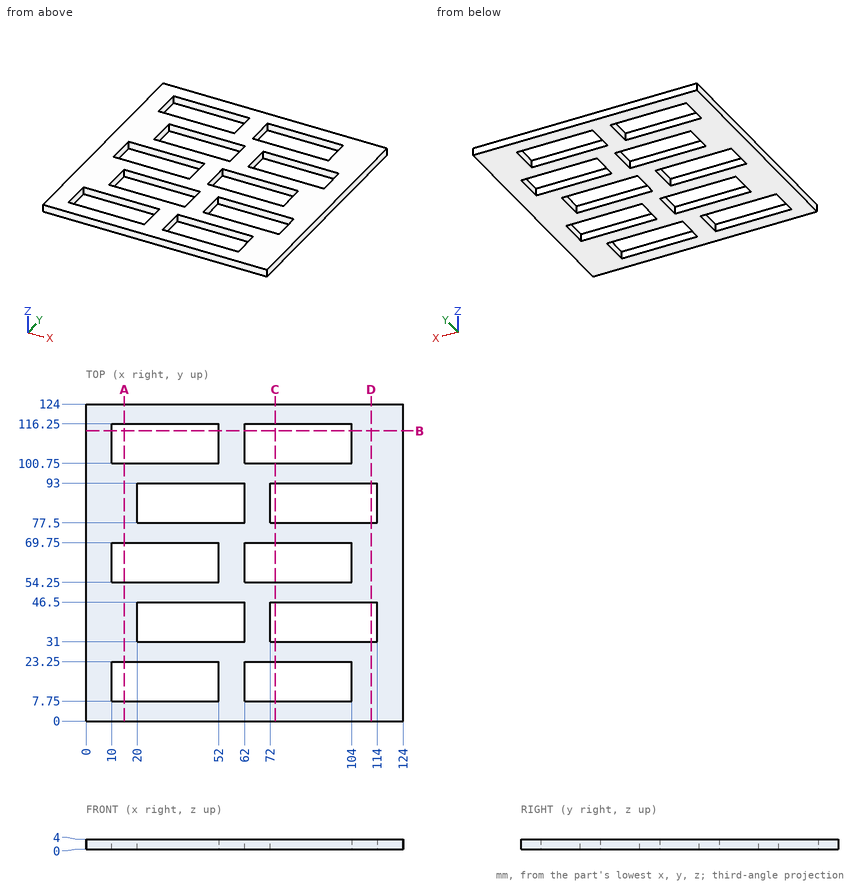
The figure shows three views and two pictorial views of one solid part (mm, origin at its lowest corner). Answer the questions. Coordinates: 2 decimals unless noted, no trailing zeros. Write each loop counter-clockwise with the first axis right and the second up, starting at its lowest first coordinate (ties: lowest second). Pieces come first, ordered by that corner, then holes. Notation, with made-up numbers: M 79.25,38.5 L 135.25,38.5 A21 ccw 135.25,76.5 Z; hole C 33,21.5 d10. An arc over 180 degrees is marked long. Answer as CSV lines item,"result". Start each with the question number.
Item 1: A flat-ended cylindrical pin translates along its axis: P1, Ø5, axis at x = 34, y = 103.5, coming from the +Z side. Find the tip coordinate at first contact, or state that the pin passes through.
Item 2: Section C-C on x = 74 is taken. Write down the section's boundary in (y, z), and give its area (3 significant figures).
Item 3: Section D-D on x = 111.5 is taken. Write down the section's boundary in (y, z), and give its area (3 significant figures).
Item 4: Section A-A on x = 15 is taken. Write down the section's boundary in (y, z).
Item 5: Consider L1, parallel to X at y = 34.5, z = 3.25; L2, parallel to Y at x = 19, z = 0.4; L3, parallel to X at y = 107, z = 1. Determine where each line is inside the solid, lowest interval first.
Item 6: Section B-B on y = 113.5 is taken. Write down the section's boundary in (x, z), and give its area (3 significant figures).
Checks:
1,P1,"passes through"
2,outline,"M 0,0 L 7.75,0 L 7.75,4 L 0,4 Z; M 23.25,0 L 31,0 L 31,4 L 23.25,4 Z; M 46.5,0 L 54.25,0 L 54.25,4 L 46.5,4 Z; M 69.75,0 L 77.5,0 L 77.5,4 L 69.75,4 Z; M 93,0 L 100.75,0 L 100.75,4 L 93,4 Z; M 116.25,0 L 124,0 L 124,4 L 116.25,4 Z"
2,area,"186 mm²"
3,outline,"M 0,0 L 31,0 L 31,4 L 0,4 Z; M 46.5,0 L 77.5,0 L 77.5,4 L 46.5,4 Z; M 93,0 L 124,0 L 124,4 L 93,4 Z"
3,area,"372 mm²"
4,outline,"M 0,0 L 7.75,0 L 7.75,4 L 0,4 Z; M 23.25,0 L 54.25,0 L 54.25,4 L 23.25,4 Z; M 69.75,0 L 100.75,0 L 100.75,4 L 69.75,4 Z; M 116.25,0 L 124,0 L 124,4 L 116.25,4 Z"
5,L1,"x = 0 to 20, 62 to 72, 114 to 124"
5,L2,"y = 0 to 7.75, 23.25 to 54.25, 69.75 to 100.75, 116.25 to 124"
5,L3,"x = 0 to 10, 52 to 62, 104 to 124"
6,outline,"M 0,0 L 10,0 L 10,4 L 0,4 Z; M 52,0 L 62,0 L 62,4 L 52,4 Z; M 104,0 L 124,0 L 124,4 L 104,4 Z"
6,area,"160 mm²"
